Job drawing, mm, ordinate dimensions from the low corner. One solid piece. A direction names the side the tool comes from. Round coordinates to 2 decimals unless told otherwise and drop trailing zeros. Write each loop counter-clockwise with the first axis right and the second up, starting at its lowest first coordinate (ties: lowest second). Pieces come first, ordered by that corner, then holes. Notation, with made-up numbers: M 40.5,20 L 47.5,20 A17 cw 47.5,46 Z; hole C 21.5,46.25 d7. An arc over 180 degrees is marked long. Answer as a JSON object with one key per item and string values. Group by question number.
1. Band-saw the part on B-B, the plane z = 1.8. Write the cut outline in (x, y).
2. Two-plate mould, pull along Z, no slides. Class the marked faces 1, 2 and 3: +Z half, -Z half, draft (parallel to the pull), parting line (faces both ways), or undercut.
3. Drill centre lines: line 1 (Z direction, x = 8, y = 12.5); line 2 (Z direction, x = 8.5, y = 14); line 3 (X direction, y = 13, z = 0.5). Where is each one in solid material? Low to high. Write a range as from..to.
4. Drop flat-ended pins along their axis: pin 1 (1 mm diameter, centred on y = 5.5, z = 3.5, fed in from +X); pin 2 (5 mm diameter, centred on x = 2, y = 4, fed in from +Z); pin 3 (1.5 mm diameter, centred on x = 8, z = 2.5, fed in from -Y). Give the stop position or say it passes through.
5. Band-saw the part on C-C, the plane z = 3.7. Write the cut outline in (x, y).
6. Which spindle directions (+Z, -Z, +X, -X, +Y, -Y) get a long thin tool onto all of the face, cutting with end or side? Do the marked faces 4 and 5. Say none if no direction does.
7. Band-saw the part on A-A, the plane x = 8. Write the cut outline in (y, z).
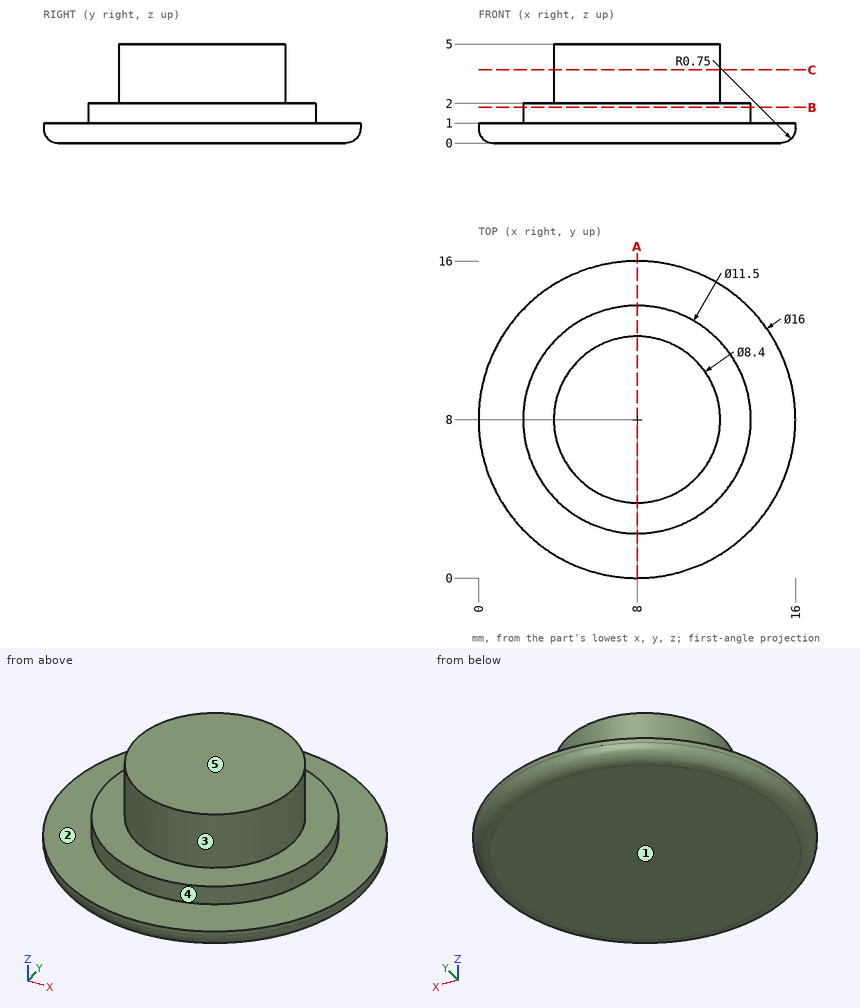
Worked answers:
{
 "1": {"outline": "C 8,8 d11.5"},
 "2": {"face 1": "-Z half", "face 2": "+Z half", "face 3": "draft"},
 "3": {"line 1": "z = 0..2", "line 2": "z = 0..1", "line 3": "x = 1.81..14.19"},
 "4": {"pin 1": "stops at x = 11.69", "pin 2": "stops at z = 2", "pin 3": "stops at y = 2.25"},
 "5": {"outline": "C 8,8 d8.4"},
 "6": {"face 4": "+Z", "face 5": "+Z, +X, -X, +Y, -Y"},
 "7": {"outline": "M 0,0.75 A0.75 ccw 0.75,0 L 15.25,0 A0.75 ccw 16,0.75 L 16,1 L 13.75,1 L 13.75,2 L 12.2,2 L 12.2,5 L 3.8,5 L 3.8,2 L 2.25,2 L 2.25,1 L 0,1 Z"}
}
